Design review of the part built by this model. Coordinates are the model's own, in mm. Round coordinates to 2 decimals unless told otherwise and drop trailing zeros. Loops run counter-clockwise (first coordinate to the right, second up) from the corner with the lowest first, then second, coordinate; pieces in that order, holes last. Notation, with made-up numbers: (-31.75, 36) - (11.25, 36) arc R22 cw to (11.25, 49) - close; hole circle Ø8 at (80, 17.25). An arc over 180 degrees is marked (long way). Return JSON: item names as keys, results as strings. Group by question number.
(1) The part is to be moulded in two halves that separate along Y. For faces 1 (the flat face through (-1, -22.5, 3)), 2 (the cylindrical face through (6.446, 10.11, 2.958)), 3 (the flat face through (-2, 15, 6)), 4 (the cylindrical face through (110, 0, 3)), say which applies: pulls with the +Y half, pulls with the -Y half, needs draft (parallel to the pull), parting line crosses it, or undercut.
(2) Wall thickness on L1, parallel to X at y = -1, z = 3.8; L2, parallel to Y at x = -87.5, z = 4.1; L3, parallel to X at y = 7.5, z = 4.65: over which ranges is each line inside the solid? List them lowest first. Write a range as [from, to].
(3) We need section C-C, the plane z = 3.55. Write out the cut boundary in (x, y), and give its area (3 significant figures).
(4) We need section A-A, the plane x = 0. Write out the cut boundary in (y, z).
(5) Clearance check with a flat-ended pin moving along its axis: pin 1 (2 mm diameter, centred on y = 10, z = 1.5, fed in from +X). State where the tip first meets the part, or that it passes through.
(6) We need section B-B, the plane y = 0. Write out the cut boundary in (x, z).
(7) We need section D-D, the plane x = -79. Write out the cut boundary in (y, z).
from build123d import *

# Parameters (mm, degrees)
SKETCH2_R           = 11.99
BOSS_EXTRUDE1_DEPTH = 6


with BuildPart() as part:
    # Sketch2 → Boss-Extrude1 (new body)
    with BuildSketch(Plane.XY):
        with BuildLine():
            Line((-87.5, -22.5), (87.5, -22.5))
            ThreePointArc((87.5, -22.5), (110, 0), (87.5, 22.5))
            Line((87.5, 22.5), (-87.5, 22.5))
            ThreePointArc((-87.5, 22.5), (-110, 0), (-87.5, -22.5))
        make_face()
        with Locations((-87.5, 0)):
            Circle(SKETCH2_R, mode=Mode.SUBTRACT)
        with Locations(Location((87.5, 0, 0), (0, 0, 180))):
            Circle(SKETCH2_R, mode=Mode.SUBTRACT)
        Circle(SKETCH2_R, mode=Mode.SUBTRACT)
    extrude(amount=BOSS_EXTRUDE1_DEPTH)


solid = part.part
Solutions:
{
 "1": {"face 1": "pulls with the -Y half", "face 2": "undercut", "face 3": "needs draft", "face 4": "parting line crosses it"},
 "2": {"L1": "[-109.98, -99.45], [-75.55, -11.95], [11.95, 75.55], [99.45, 109.98]", "L2": "[-22.5, -11.99], [11.99, 22.5]", "L3": "[-108.71, -96.85], [-78.15, -9.35], [9.35, 78.15], [96.85, 108.71]"},
 "3": {"outline": "(-87.5, -22.5) - (87.5, -22.5) arc R22.5 ccw to (87.5, 22.5) - (-87.5, 22.5) arc R22.5 ccw to start; hole circle Ø23.98 at (-87.5, 0); hole circle Ø23.98 at (0, 0); hole circle Ø23.98 at (87.5, 0)", "area": "8,110 mm^2"},
 "4": {"outline": "(-22.5, 0) - (-11.99, 0) - (-11.99, 6) - (-22.5, 6) - close; (11.99, 0) - (22.5, 0) - (22.5, 6) - (11.99, 6) - close"},
 "5": {"pin 1": "x = 108.12"},
 "6": {"outline": "(-110, 0) - (-99.49, 0) - (-99.49, 6) - (-110, 6) - close; (-75.51, 0) - (-11.99, 0) - (-11.99, 6) - (-75.51, 6) - close; (11.99, 0) - (75.51, 0) - (75.51, 6) - (11.99, 6) - close; (99.49, 0) - (110, 0) - (110, 6) - (99.49, 6) - close"},
 "7": {"outline": "(-22.5, 0) - (-8.46, 0) - (-8.46, 6) - (-22.5, 6) - close; (8.46, 0) - (22.5, 0) - (22.5, 6) - (8.46, 6) - close"}
}
